```python
from build123d import *

# Parameters (mm, degrees)
SKETCH033_W     = 12.4
SKETCH033_H     = 12.4
PAD015_DEPTH    = 5.8
PAD016_DEPTH    = 2.6
SKETCH035_R     = 3
POCKET010_DEPTH = 0.6
SKETCH036_R     = 4
POCKET011_DEPTH = 2
CHAMFER_SIZE    = 0.4
FILLET_R        = 0.6


with BuildPart() as part:
    # Sketch033 → Pad015 (new body)
    with BuildSketch(Plane.XY):
        Rectangle(SKETCH033_W, SKETCH033_H)
    extrude(amount=PAD015_DEPTH)

    # Sketch034 (on Face6 of Pad015) → Pad016 (join)
    with BuildSketch(Plane.XY.offset(5.8)):
        with BuildLine():
            Line((-4.5, 5.5), (4.5, 5.5))
            ThreePointArc((5.5, 4.5), (5.207107, 5.207107), (4.5, 5.5))
            Line((5.5, 4.5), (5.5, -4.5))
            ThreePointArc((4.5, -5.5), (5.207107, -5.207107), (5.5, -4.5))
            Line((4.5, -5.5), (-4.5, -5.5))
            ThreePointArc((-5.5, -4.5), (-5.207107, -5.207107), (-4.5, -5.5))
            Line((-5.5, -4.5), (-5.5, 4.5))
            ThreePointArc((-4.5, 5.5), (-5.207107, 5.207107), (-5.5, 4.5))
        make_face()
    extrude(amount=PAD016_DEPTH)

    # Sketch035 (on Face15 of Pad016) → Pocket010 (cut)
    with BuildSketch(Plane.XY.offset(8.4)):
        Circle(SKETCH035_R)
    extrude(amount=-POCKET010_DEPTH, mode=Mode.SUBTRACT)

    # Sketch036 (on Face4 of Pocket010) → Pocket011 (cut)
    with BuildSketch(Plane(origin=(0, 0, 0), x_dir=(1, 0, 0), z_dir=(0, 0, -1))):
        Circle(SKETCH036_R)
    extrude(amount=-POCKET011_DEPTH, mode=Mode.SUBTRACT)

    # Chamfer
    chamfer_edges = [part.edges().sort_by_distance(p)[0] for p in [
        (-3, 0, 8.4),
    ]]
    chamfer(chamfer_edges, length=CHAMFER_SIZE)

    # Fillet
    fillet_edges = [part.edges().sort_by_distance(p)[0] for p in [
        (0, -5.5, 8.4),
        (-5.207107, -5.207107, 8.4),
        (-5.5, 0, 8.4),
        (-5.207107, 5.207107, 8.4),
        (0, 5.5, 8.4),
        (-3.4, 0, 8.4),
        (5.207107, -5.207107, 8.4),
        (5.207107, 5.207107, 8.4),
        (5.5, 0, 8.4),
    ]]
    fillet(fillet_edges, radius=FILLET_R)


with BuildPart() as part_1:
    # Body004 placement: moved
    add(part.part.moved(Location((-4.6, -39.7, 15.8))))


solid = part_1.part
```
The listing builds one solid part. Answer for the finished solid, in the listing's coordinates (mm). A direction names the side the tool comes from. Round coordinates to 2 decimals unless told otherwise and drop trailing zeros. Loops run counter-clockwise (first coordinate to the right, second up) from the corner with the lowest first, then second, coordinate; pieces in that order, holes last. Notation, with made-up numbers: (53, 0) - (106, 0) arc R27 ccw to (106, 32) - close; hole circle Ø1 at (-39, 10.5). An arc over 180 degrees is marked (long way). Use one line per item in the form item = value. Start each with the question number.
1. The part is cut by section A-A on y = -39.7. Determine the outline of the cut face in (x, z), then the cut area to 3 significant figures.
2. A tool of negligible diameter and unlimited length cuts with its end or side. For faces 1 (the face through (-5.467, -35.795, 16.786)), 2 (the face through (-5, -40, 23.6)), 3 (the face through (0.615, -34.501, 22.586)), 4 (the face through (0.599, -44.915, 22.586)), from which of +Z, -Z, +X, -X, +Y, -Y can it reach the whole face along a straight path? Write none if from no direction.
3. Consider line 1 (X direction, y = -39.7, z = 16.8); line 2 (Y direction, x = -4.6, z = 17.2); line 3 (Z direction, x = -5, y = -36.5). Determine where each line is inside the solid, lowest interval first. Write a range as [from, to].
4. The part is cut by section B-B on z = 17. Determine the outline of the cut face in (x, y), then the cut area to 3 significant figures.
5. The part is cut by section C-C on x = -4.6. Determine the outline of the cut face in (y, z), then the cut area to 3 significant figures.
6. Given pin 1 Ø5 at (x, y) = (-4.6, -39.7) entering from -Z; pin 2 Ø0.6 at (x, z) = (-5.5, 22.5) entering from +Y; pin 3 Ø2 at (y, z) = (-39.5, 23) entering from -X, each flat-ended and moving along its own axis, determine where each tip first touches the part or whether it passes through.
7. For a pull along X with two mould halves and no side action, classify faces 5 (the face through (-5, -45.9, 19)), 6 (the face through (-5, -40, 17.8)), 7 (the face through (-9.815, -44.899, 22.586)) as pulls with the +X half, pulls with the -X half, needs draft (parallel to the pull), parting line crosses it, or undercut.
Geometry check:
q1.outline = (-10.8, 15.8) - (-8.6, 15.8) - (-8.6, 17.8) - (-0.6, 17.8) - (-0.6, 15.8) - (1.6, 15.8) - (1.6, 21.6) - (0.9, 21.6) - (0.9, 23.6) arc R0.6 ccw to (0.3, 24.2) - (-0.95, 24.2) arc R0.6 ccw to (-1.38, 24.02) - (-1.6, 23.8) - (-1.6, 23.6) - (-7.6, 23.6) - (-7.6, 23.8) - (-7.82, 24.02) arc R0.6 ccw to (-8.25, 24.2) - (-9.5, 24.2) arc R0.6 ccw to (-10.1, 23.6) - (-10.1, 21.6) - (-10.8, 21.6) - close
q1.area = 80.6 mm^2
q2.face_1 = -Z
q2.face_2 = +Z
q2.face_3 = +Z, +X, +Y
q2.face_4 = +Z, +X, -Y
q3.line_1 = [-10.8, -8.6], [-0.6, 1.6]
q3.line_2 = [-45.9, -43.7], [-35.7, -33.5]
q3.line_3 = [17.8, 24.02]
q4.outline = (-10.8, -45.9) - (1.6, -45.9) - (1.6, -33.5) - (-10.8, -33.5) - close; hole circle Ø8 at (-4.6, -39.7)
q4.area = 103 mm^2
q5.outline = (-45.9, 15.8) - (-43.7, 15.8) - (-43.7, 17.8) - (-35.7, 17.8) - (-35.7, 15.8) - (-33.5, 15.8) - (-33.5, 21.6) - (-34.2, 21.6) - (-34.2, 23.6) arc R0.6 ccw to (-34.8, 24.2) - (-36.05, 24.2) arc R0.6 ccw to (-36.48, 24.02) - (-36.7, 23.8) - (-36.7, 23.6) - (-42.7, 23.6) - (-42.7, 23.8) - (-42.92, 24.02) arc R0.6 ccw to (-43.35, 24.2) - (-44.6, 24.2) arc R0.6 ccw to (-45.2, 23.6) - (-45.2, 21.6) - (-45.9, 21.6) - close
q5.area = 80.6 mm^2
q6.pin_1 = 17.8
q6.pin_2 = -34.2
q6.pin_3 = -10.1
q7.face_5 = needs draft
q7.face_6 = undercut
q7.face_7 = pulls with the -X half
